Here's how the part is built. I have some questions about the finished solid (model axes, mm). Face numbers are marked on the shaded views. A direction names the side the tool comes from. Coordinates: 2 decimals unless noted, no trailing zeros. Order: outer loops, then holes, each group sorted by start corner. A loop starts at its lowest first (then second) coordinate and runs counter-clockwise, first axis right, second up.
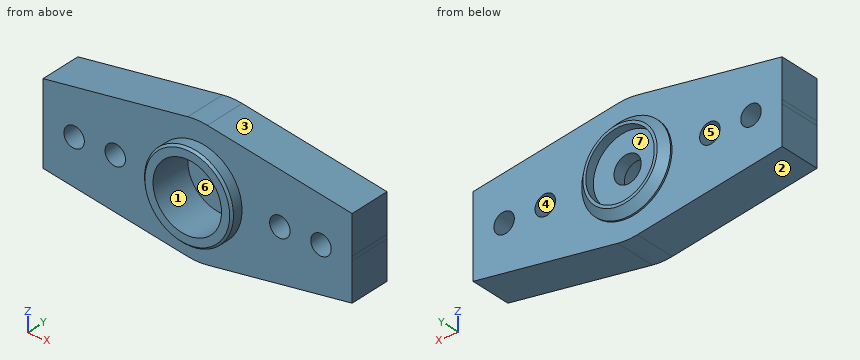
```python
from build123d import *

# Parameters (mm, degrees)
SKETCH1_R           = 1.651
SKETCH1_R_2         = 1.2446
BOSS_EXTRUDE1_DEPTH = 5.08
SKETCH2_R           = 5.40385
SKETCH2_R_2         = 4.1656
BOSS_EXTRUDE2_DEPTH = 1.0922
CHAMFER1_SIZE       = 0.889
SKETCH4_R           = 5.4102
SKETCH4_R_2         = 4.1656
BOSS_EXTRUDE3_DEPTH = 1.4986
CHAMFER2_SIZE       = 0.254
SKETCH5_W           = 15.127715844
SKETCH5_H           = 12.166577881
CUT_EXTRUDE1_DEPTH  = 7.5786
SKETCH6_R           = 4.1656
CUT_EXTRUDE2_DEPTH  = 3.556


with BuildPart() as part:
    # Sketch1 → Boss-Extrude1 (new body)
    with BuildSketch(Plane(origin=(0, 0, 0), x_dir=(1, 0, 0), z_dir=(0, 1, 0))):
        with BuildLine():
            Line((-30.503852792, 3.086942476), (-1.192854484, 7.654613457))
            ThreePointArc((-1.192854484, 7.654613457), (0, 7.747), (1.192854484, 7.654613457))
            Line((1.192854484, 7.654613457), (30.503852792, 3.086942476))
            ThreePointArc((30.503852792, 3.086942476), (33.147, 0), (30.503852792, -3.086942476))
            Line((30.503852792, -3.086942476), (1.192854484, -7.654613457))
            ThreePointArc((1.192854484, -7.654613457), (0, -7.747), (-1.192854484, -7.654613457))
            Line((-1.192854484, -7.654613457), (-30.503852792, -3.086942476))
            ThreePointArc((-30.503852792, -3.086942476), (-33.147, 0), (-30.503852792, 3.086942476))
        make_face()
        Circle(SKETCH1_R, mode=Mode.SUBTRACT)
        with Locations((-10.0076, 0)):
            Circle(SKETCH1_R_2, mode=Mode.SUBTRACT)
        with Locations((-15.0114, 0)):
            Circle(SKETCH1_R_2, mode=Mode.SUBTRACT)
        with Locations((-20.0152, 0)):
            Circle(SKETCH1_R_2, mode=Mode.SUBTRACT)
        with Locations((-25.019, 0)):
            Circle(SKETCH1_R_2, mode=Mode.SUBTRACT)
        with Locations((-30.0228, 0)):
            Circle(SKETCH1_R_2, mode=Mode.SUBTRACT)
        with Locations((30.0228, 0)):
            Circle(SKETCH1_R_2, mode=Mode.SUBTRACT)
        with Locations((25.019, 0)):
            Circle(SKETCH1_R_2, mode=Mode.SUBTRACT)
        with Locations((20.0152, 0)):
            Circle(SKETCH1_R_2, mode=Mode.SUBTRACT)
        with Locations((15.0114, 0)):
            Circle(SKETCH1_R_2, mode=Mode.SUBTRACT)
        with Locations((10.0076, 0)):
            Circle(SKETCH1_R_2, mode=Mode.SUBTRACT)
    extrude(amount=BOSS_EXTRUDE1_DEPTH)

    # Sketch2 → Boss-Extrude2 (add)
    with BuildSketch(Plane(origin=(0, 5.08, 0), x_dir=(1, 0, 0), z_dir=(0, 1, 0))):
        Circle(SKETCH2_R)
        Circle(SKETCH2_R_2, mode=Mode.SUBTRACT)
    extrude(amount=BOSS_EXTRUDE2_DEPTH)

    # Chamfer1
    chamfer1_edges = [part.edges().sort_by_distance(p)[0] for p in [
        (-5.40385, 6.1722, 0),
    ]]
    chamfer(chamfer1_edges, length=CHAMFER1_SIZE)

    # Sketch4 → Boss-Extrude3 (add)
    with BuildSketch(Plane.XZ):
        Circle(SKETCH4_R)
        Circle(SKETCH4_R_2, mode=Mode.SUBTRACT)
    extrude(amount=BOSS_EXTRUDE3_DEPTH)

    # Chamfer2
    chamfer2_edges = [part.edges().sort_by_distance(p)[0] for p in [
        (-5.4102, -1.4986, 0),
    ]]
    chamfer(chamfer2_edges, length=CHAMFER2_SIZE)

    # Sketch5 → Cut-Extrude1 (cut, through all)
    with BuildSketch(Plane(origin=(0, 5.08, 0), x_dir=(1, 0, 0), z_dir=(0, 1, 0))):
        with Locations((-26.359857922, -0.574807794)):
            Rectangle(SKETCH5_W, SKETCH5_H)
        with Locations((26.359857922, -0.574807794)):
            Rectangle(SKETCH5_W, SKETCH5_H)
    extrude(amount=-CUT_EXTRUDE1_DEPTH, mode=Mode.SUBTRACT)

    # Sketch6 → Cut-Extrude2 (cut)
    with BuildSketch(Plane.XZ):
        Circle(SKETCH6_R)
    extrude(amount=-CUT_EXTRUDE2_DEPTH, mode=Mode.SUBTRACT)


solid = part.part
```
Q1. I need wall thicknesses on L1, parallel to Y at x = -1, z = 2.5; L2, parallel to Y at x = -16, z = 2; L3, parallel to Z at x = 0, y = 5.4. Which ranges of each line are inside material? Lowest first, please.
Q2. If we section it at A-A on x = 0: Write out the boundary of the cut face in (y, z).
Q3. We'd pull the mould along X, two halves only. Please class the marked faces 1, 2, 3 and 4: pulls with the +X half, pulls with the -X half, needs draft (parallel to the pull), parting line crosses it, or undercut.
Q4. For the marked faces 5, 6 and 7, which set-ups out of +Z, -Z, +X, -X, +Y, -Y let a thin tool reach every point of the face, with its end or its side?
Q5. Will these pins go through, and if not, where does the flat tip stop? pin 1 (2.5 mm diameter, centred on x = -0.5, z = -0.5, fed in from +Y); pin 2 (6.5 mm diameter, centred on x = 0, z = 0, fed in from -Y); pin 3 (4 mm diameter, centred on x = 8.5, y = 5, fed in from +Z); pin 4 (2 mm diameter, centred on x = 15.01, z = 0, fed in from -Y).
Q6. If we section it at B-B on y = 2.25: Write out the boundary of the cut face in (x, z).
Q7. If we section it at C-C on y = -0.5: Write out the boundary of the cut face in (x, z).
Q8. If we section it at D-D on x = 7.5: Write out the boundary of the cut face in (y, z), then the cut area to 3 significant figures.
Reply:
1. L1: y = 3.56 to 5.08
1. L2: y = 0 to 5.08
1. L3: z = -5.29 to -4.17, 4.17 to 5.29
2. outline: (-1.5, -5.16) - (-1.24, -5.41) - (0, -5.41) - (0, -7.75) - (5.08, -7.75) - (5.08, -5.4) - (5.28, -5.4) - (6.17, -4.51) - (6.17, -4.17) - (5.08, -4.17) - (5.08, -1.65) - (3.56, -1.65) - (3.56, -4.17) - (-1.5, -4.17) - close; (-1.5, 4.17) - (3.56, 4.17) - (3.56, 1.65) - (5.08, 1.65) - (5.08, 4.17) - (6.17, 4.17) - (6.17, 4.51) - (5.28, 5.4) - (5.08, 5.4) - (5.08, 7.75) - (0, 7.75) - (0, 5.41) - (-1.24, 5.41) - (-1.5, 5.16) - close
3. face 1: undercut
3. face 2: pulls with the -X half
3. face 3: pulls with the +X half
3. face 4: undercut
4. face 5: +Y, -Y
4. face 6: -Y
4. face 7: +Y
5. pin 1: stops at y = 5.08
5. pin 2: stops at y = 3.56
5. pin 3: stops at z = 6.83
5. pin 4: passes through
6. outline: (-18.8, -4.91) - (-1.19, -7.65) arc R7.75 ccw to (1.19, -7.65) - (18.8, -4.91) - (18.8, -0.25) arc R1.24 cw to (18.8, 0.25) - (18.8, 4.91) - (1.19, 7.65) arc R7.75 ccw to (-1.19, 7.65) - (-18.8, 4.91) - (-18.8, 0.25) arc R1.24 cw to (-18.8, -0.25) - close; hole circle Ø2.49 at (-15.01, 0); hole circle Ø2.49 at (-10.01, 0); hole circle Ø8.33 at (0, 0); hole circle Ø2.49 at (10.01, 0); hole circle Ø2.49 at (15.01, 0)
7. outline: circle Ø10.82 at (0, 0); hole circle Ø8.33 at (0, 0)
8. outline: (0, -6.67) - (5.08, -6.67) - (5.08, 6.67) - (0, 6.67) - close
8. area: 67.8 mm2
